from build123d import *

# Parameters (mm, degrees)
SKETCH1_W                 = 30
SKETCH1_H                 = 30
BOSS_EXTRUDE1_DEPTH       = 30
CUT_EXTRUDE1_START        = -31
CUT_EXTRUDE1_DEPTH        = 32
SKETCH3_OUTSIDE_W         = 42.392
SKETCH3_OUTSIDE_H         = 42.392
SKETCH3_OUTSIDE_W_2       = 2
SKETCH3_OUTSIDE_H_2       = 2
CUT_EXTRUDE2_DEPTH        = 1
F_8_32_TAPPED_HOLE1_D     = 3.4544
F_8_32_TAPPED_HOLE1_DEPTH = 10.7188
F_8_32_TAPPED_HOLE1_TIP   = 1.037806461
F_4_40_TAPPED_HOLE1_D     = 2.2606
F_4_40_TAPPED_HOLE1_DEPTH = 7.5946
F_4_40_TAPPED_HOLE1_TIP   = 0.679152758
FILLET1_R                 = 1.000000032
CHAMFER1_SIZE             = 0.5


with BuildPart() as part:
    # Sketch1 → Boss-Extrude1 (new body)
    with BuildSketch(Plane(origin=(0, 0, 0), x_dir=(1, 0, 0), z_dir=(0, 1, 0))):
        Rectangle(SKETCH1_W, SKETCH1_H)
    extrude(amount=BOSS_EXTRUDE1_DEPTH)

    # Sketch2 → Cut-Extrude1 (cut)
    with BuildSketch(Plane(origin=(0, 30, 0), x_dir=(1, 0, 0), z_dir=(0, 1, 0)).offset(CUT_EXTRUDE1_START)):
        with BuildLine():
            Line((97.111025509, 5), (15, 5))
            ThreePointArc((15, 5), (7.928932188, 7.928932188), (5, 15))
            Line((5, 15), (5, 97.111025509))
            Line((5, 97.111025509), (121.122525896, 213.233551405))
            Line((121.122525896, 213.233551405), (213.233551405, 121.122525896))
            Line((213.233551405, 121.122525896), (97.111025509, 5))
        make_face()
    cut_extrude1 = extrude(amount=CUT_EXTRUDE1_DEPTH, mode=Mode.SUBTRACT)

    # Mirror1: Cut-Extrude1 across plane
    add(cut_extrude1.mirror(Plane.XY), mode=Mode.SUBTRACT)

    # Sketch3 outside → Cut-Extrude2 (cut)
    with BuildSketch(Plane.XZ):
        Rectangle(SKETCH3_OUTSIDE_W, SKETCH3_OUTSIDE_H)
        with Locations((-14, 14)):
            Rectangle(SKETCH3_OUTSIDE_W_2, SKETCH3_OUTSIDE_H_2, mode=Mode.SUBTRACT)
        with Locations((-14, -14)):
            Rectangle(SKETCH3_OUTSIDE_W_2, SKETCH3_OUTSIDE_H_2, mode=Mode.SUBTRACT)
        with Locations((14, 0)):
            Rectangle(SKETCH3_OUTSIDE_W_2, SKETCH3_OUTSIDE_H_2, mode=Mode.SUBTRACT)
    extrude(amount=-CUT_EXTRUDE2_DEPTH, mode=Mode.SUBTRACT)

    # #8-32 Tapped Hole1
    with Locations(Plane.XZ.offset(-1)):
        with Locations((0, 0)):
            Hole(F_8_32_TAPPED_HOLE1_D / 2, depth=F_8_32_TAPPED_HOLE1_DEPTH)
            with Locations((0, 0, -(F_8_32_TAPPED_HOLE1_DEPTH + F_8_32_TAPPED_HOLE1_TIP / 2))):  # 118° drill point
                Cone(0, F_8_32_TAPPED_HOLE1_D / 2, F_8_32_TAPPED_HOLE1_TIP, mode=Mode.SUBTRACT)

    # #4-40 Tapped Hole1
    with Locations(Plane(origin=(0, 30, 0), x_dir=(-1, 0, 0), z_dir=(0, 1, 0))):
        with Locations((0, 0)):
            Hole(F_4_40_TAPPED_HOLE1_D / 2, depth=F_4_40_TAPPED_HOLE1_DEPTH)
            with Locations((0, 0, -(F_4_40_TAPPED_HOLE1_DEPTH + F_4_40_TAPPED_HOLE1_TIP / 2))):  # 118° drill point
                Cone(0, F_4_40_TAPPED_HOLE1_D / 2, F_4_40_TAPPED_HOLE1_TIP, mode=Mode.SUBTRACT)

    # Fillet1
    fillet1_edges = [part.edges().sort_by_distance(p)[0] for p in [
        (-15, 15, 15),
        (-15, 15, -15),
    ]]
    fillet(fillet1_edges, radius=FILLET1_R)

    # Chamfer1
    chamfer1_edges = [part.edges().sort_by_distance(p)[0] for p in [
        (-14.707106772, 30, -14.707106772),
        (-14.707106772, 30, 14.707106772),
        (-4.499999984, 30, -15),
        (7.928932188, 30, -7.928932188),
        (7.928932188, 30, 7.928932188),
        (-4.499999984, 30, 15),
        (-15, 30, 0),
    ]]
    chamfer(chamfer1_edges, length=CHAMFER1_SIZE)


solid = part.part
The listing builds one solid part. Answer for the finished solid, in the listing's coordinates (mm). A direction names the side the tool comes from. Round coordinates to 2 decimals unless told otherwise and drop trailing zeros. Write each loop counter-clockwise with the first axis right and the second up, starting at its lowest first coordinate (ties: lowest second). Pieces come first, ordered by that corner, then holes. Notation, with made-up numbers: M 59.5,38 L 83.5,38 A28 ccw 83.5,72 Z; hole C 54,-37.75 d6. An arc over 180 degrees is marked long. Write each question's results on one line, items separated by ' | '. Start each with the question number.
Item 1: Which of the six approach directions +Z, -Z, +X, -X, +Y, -Y give full straight-line access (tool end or side, diameter ignored) to faces 4 (the flat face through (13, 0.5, 0)), 5 (the flat face through (14, 0.5, 1)), 6 (the flat face through (-14, 0.5, 13))?
Item 2: Find section A-A on y = 10. Write down the section's boundary in (x, z).
Item 3: Find section C-C on x = -7.25. Write down the section's boundary in (y, z).
Item 4: Given pin 1 Ø0.8 at (x, y) = (13.5, 0.5) entering from -Z; pin 2 Ø1.1 at (y, z) = (0.5, -13.5) entering from +X; pin 3 Ø1.4 at (x, z) = (0, 0) entering from -Y, each flat-ended and moving along its own axis, determine where each tip first touches the part or whether it passes through.
Item 5: The mould has two halves that part along X. Classify faces 1 (the flat face through (-5, 15, -15)), 2 (the conical face through (0.277, 12.576, -0.115)), 3 (the cylindrical face through (-14.715, 14.956, 14.699)): +X half, -X half, draft (parallel to the pull), parting line (faces both ways), or undercut.
Item 6: Straight lines are drawn through the part: probe 1 along Z at (x, y) = (0, 26.5); probe 2 along Z at (x, y) = (0, 3.5). For each, find the intervals that lie inside material, in ascending order.
Item 7: Find section D-D on z = 4. Write down the section's boundary in (x, y).
Item 8: Find section B-B on y = 13.5. Write down the section's boundary in (x, z).
Answer block:
1) face 4: +Z, -Z, -X, -Y | face 5: +Z, +X, -X, -Y | face 6: +X, -X, -Y
2) outline: M -15,-14 A1 ccw -14,-15 L 5,-15 A10 cw 15,-5 L 15,5 A10 cw 5,15 L -14,15 A1 ccw -15,14 Z; hole C 0,0 d3.45
3) outline: M 1,-15 L 29.5,-15 L 30,-14.5 L 30,14.5 L 29.5,15 L 1,15 Z
4) pin 1: stops at z = -1 | pin 2: stops at x = 5.15 | pin 3: stops at y = 12.34
5) face 1: draft | face 2: undercut | face 3: -X half
6) probe 1: z = -15 to -1.13, 1.13 to 15 | probe 2: z = -15 to -1.73, 1.73 to 15
7) outline: M -15,1 L 15,1 L 15,30 L -14.5,30 L -15,29.5 Z
8) outline: M -15,-14 A1 ccw -14,-15 L 5,-15 A10 cw 15,-5 L 15,5 A10 cw 5,15 L -14,15 A1 ccw -15,14 Z
